Input: dimensioned drawing with shaded views. Units: mm. Origin: part minimum x, y, z. A direction names the side the tool comes from. Round coordinates to 2 decimals unless told otherwise and drop trailing zeros. Order: outer loops, then holes, each group sorted by start corner. A loop starts at its lowest first (then second) coordinate and runs counter-clockwise, first axis right, second up. Notation, with made-up numbers: M 21,64 L 53,64 A24 ccw 53,102 Z; hole C 53,78 d9. An arc over 180 degrees is marked long. One line per question, with ' | ' between items.
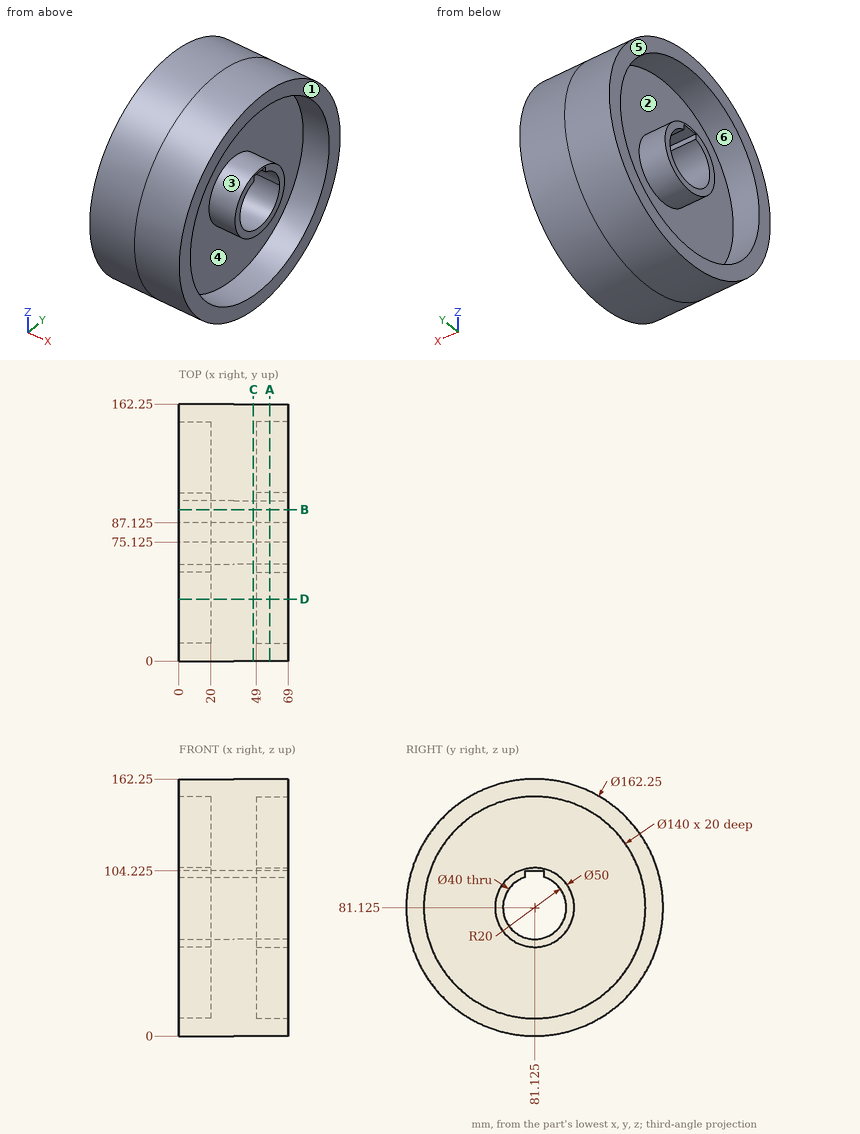
Item 1: Section query C-C, the plane x = 47. Return loops of the section in (y, z) (3 decimals), plus the area to 3 significant figures.
Report:
outline: C 81.125,81.125 d162.25; hole M 75.125,100.204 A20 ccw long 87.125,100.204 L 87.125,104.225 L 75.125,104.225 Z | area: 19,400 mm²
Item 2: Line query: line 1 along Z through (x, y) = (4, 95); line 2 along Z through (x, y) = (7.5, 61); line 3 along Z through (x, y) = (55.5, 67). Output: solid intervals per line, ascending. Write a range as from..to.
Report:
line 1: 1.2..12.51, 60.33..66.72, 95.53..101.92, 149.74..161.05 | line 2: 2.54..14.08, 66.29..95.96, 148.17..159.71 | line 3: 1.24..12.56, 60.5..66.97, 95.28..101.75, 149.69..161.01
Item 3: First-contact query: pin 1 (4.5 mm diameter, centred on x = 44, z = 102.5, fed in from +Y); pin 2 (4.5 mm diameter, centred on x = 33.5, z = 103, fed in from -Y); pin 3 (10 mm diameter, centred on y = 19.5, z = 68, fed in from +X); pin 4 (12 mm diameter, centred on y = 18.5, z = 54.5, fed in from +X). Flat tips, straight axial feed; report the tip coordinate or a pass-through.
Report:
pin 1: y = 159.96 | pin 2: y = 2.41 | pin 3: x = 49 | pin 4: x = 69
Item 4: Section query A-A, the plane x = 57.5. Return loops of the section in (y, z) (3 decimals).
Report:
outline: C 81.125,81.125 d162.25; C 81.125,81.125 d50; hole C 81.125,81.125 d140; hole M 75.125,100.204 A20 ccw long 87.125,100.204 L 87.125,104.225 L 75.125,104.225 Z
Item 5: Access query for the marked faces 1, 2 and 3. Directions: +Z, -Z, +X, -X, +Y, -Y. A direction counts if a zero-diameter tool reaches every point of the face in a straight line with its end or side. Return the directions, or none.
Report:
face 1: +Z, -Z, +X, +Y, -Y | face 2: -X | face 3: +X
Item 6: Section query B-B, the plane y = 95.5. Return loops of the section in (x, z).
Report:
outline: M 0,1.28 L 69,1.28 L 69,12.62 L 49,12.62 L 49,60.67 L 69,60.67 L 69,67.22 L 0,67.22 L 0,60.67 L 20,60.67 L 20,12.62 L 0,12.62 Z; M 0,95.03 L 69,95.03 L 69,101.58 L 49,101.58 L 49,149.63 L 69,149.63 L 69,160.97 L 0,160.97 L 0,149.63 L 20,149.63 L 20,101.58 L 0,101.58 Z
Item 7: Section query D-D, the plane y = 39. Return loops of the section in (x, z).
Report:
outline: M 0,11.79 L 69,11.79 L 69,25.22 L 49,25.22 L 49,137.03 L 69,137.03 L 69,150.46 L 0,150.46 L 0,137.03 L 20,137.03 L 20,25.22 L 0,25.22 Z
Item 8: Mould query, pull axis Y, two halves, no side actions, for the marked faces 4, 5 and 6. Classes: +Y half, -Y half, draft (parallel to the pull), parting line (faces both ways), or undercut.
Report:
face 4: undercut | face 5: draft | face 6: undercut
